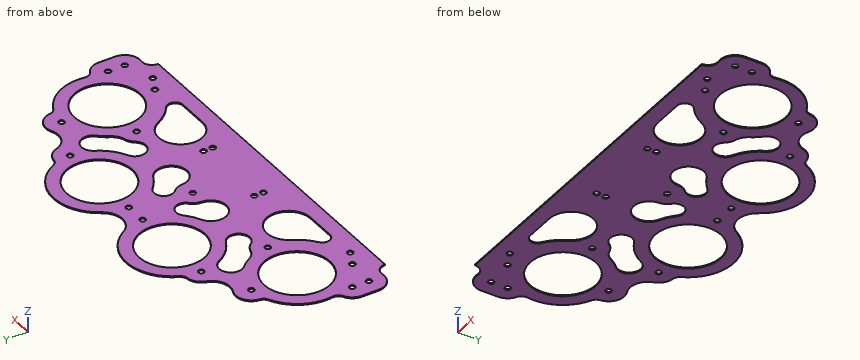
```python
from build123d import *

# Parameters (mm, degrees)
MODEL_R            = 21.5
MODEL_R_2          = 1.89865
BASE_FLANGE1_DEPTH = 0.7


# Sheet-metal steps are written as plain solids
with BuildPart() as part:
    # Model → Base-Flange1 (new body)
    with BuildSketch(Plane.XY):
        with BuildLine():
            Line((-134.72553251, -2.711313899), (-134.72553251, 8.193532943))
            ThreePointArc((-134.72553251, 8.193532943), (-133.25770932, 13.409082664), (-129.285140732, 17.093531418))
            ThreePointArc((-129.285140732, 17.093531418), (-127.122461212, 19.249115875), (-126.616601885, 22.260400219))
            ThreePointArc((-126.616601885, 22.260400219), (-123.404934832, 40.6646253), (-109.924644657, 53.599542498))
            ThreePointArc((-109.924644657, 53.599542498), (-107.998724055, 55.233004005), (-107.116719879, 57.599316598))
            ThreePointArc((-107.116719879, 57.599316598), (-101.974015213, 65.474503584), (-92.575264278, 65.83431216))
            ThreePointArc((-92.575264278, 65.83431216), (-82.894170466, 65.746450056), (-76.506575672, 73.021745919))
            ThreePointArc((-76.506575672, 73.021745919), (-73.335376859, 77.830552746), (-68.037655249, 80.092249178))
            ThreePointArc((-68.037655249, 80.092249178), (-65.683638934, 80.995038824), (-64.06940128, 82.931700578))
            ThreePointArc((-64.06940128, 82.931700578), (-38.361840541, 100.119815012), (-11.129181755, 85.467434576))
            ThreePointArc((-11.129181755, 85.467434576), (0.155495187, 79.042938382), (11.440172129, 85.467434576))
            ThreePointArc((11.440172129, 85.467434576), (38.672830915, 100.119815012), (64.380391655, 82.931700578))
            ThreePointArc((64.380391655, 82.931700578), (65.994629309, 80.995038824), (68.348645623, 80.092249178))
            ThreePointArc((68.348645623, 80.092249178), (73.646367234, 77.830552746), (76.817566047, 73.021745919))
            ThreePointArc((76.817566047, 73.021745919), (83.205160841, 65.746450057), (92.886254653, 65.83431216))
            ThreePointArc((92.886254653, 65.83431216), (102.285005587, 65.474503584), (107.427710253, 57.599316599))
            ThreePointArc((107.427710253, 57.599316599), (108.309714429, 55.233004005), (110.235635031, 53.599542498))
            ThreePointArc((110.235635031, 53.599542498), (123.715925206, 40.6646253), (126.92759226, 22.260400219))
            ThreePointArc((126.92759226, 22.260400219), (127.433451587, 19.249115875), (129.596131107, 17.093531418))
            ThreePointArc((129.596131107, 17.093531418), (133.568699694, 13.409082664), (135.036522885, 8.193532943))
            Line((135.036522885, 8.193532943), (135.036522885, -2.711313899))
            ThreePointArc((135.036522885, -2.711313899), (131.562361662, -10.288478821), (123.553837233, -12.600785232))
            ThreePointArc((123.553837233, -12.600785232), (118.393911689, -14.090613855), (116.155495187, -18.972612677))
            Line((116.155495187, -18.972612677), (-115.844504813, -18.972612677))
            ThreePointArc((-115.844504813, -18.972612677), (-118.082921315, -14.090613855), (-123.242846859, -12.600785232))
            ThreePointArc((-123.242846859, -12.600785232), (-131.251371287, -10.288478821), (-134.72553251, -2.711313899))
        make_face()
        with Locations((97.237534512, 26.561617598)):
            Circle(MODEL_R, mode=Mode.SUBTRACT)
        with Locations((37.237534512, 70.154169278)):
            Circle(MODEL_R, mode=Mode.SUBTRACT)
        with Locations((-36.926544138, 70.154169278)):
            Circle(MODEL_R, mode=Mode.SUBTRACT)
        with Locations((-96.926544138, 26.561617598)):
            Circle(MODEL_R, mode=Mode.SUBTRACT)
        with Locations((-66.926544138, 26.561617598)):
            Circle(MODEL_R_2, mode=Mode.SUBTRACT)
        with Locations((-96.926544138, 56.561617598)):
            Circle(MODEL_R_2, mode=Mode.SUBTRACT)
        with Locations((-66.926544138, 70.154169278)):
            Circle(MODEL_R_2, mode=Mode.SUBTRACT)
        with Locations((-6.926544138, 70.154169278)):
            Circle(MODEL_R_2, mode=Mode.SUBTRACT)
        with Locations((7.237534512, 70.154169278)):
            Circle(MODEL_R_2, mode=Mode.SUBTRACT)
        with Locations((67.237534512, 70.154169278)):
            Circle(MODEL_R_2, mode=Mode.SUBTRACT)
        with Locations((67.237534512, 26.561617598)):
            Circle(MODEL_R_2, mode=Mode.SUBTRACT)
        with Locations((97.237534512, 56.561617598)):
            Circle(MODEL_R_2, mode=Mode.SUBTRACT)
        with Locations((31.205495187, 5.741109522)):
            Circle(MODEL_R_2, mode=Mode.SUBTRACT)
        with Locations((31.205495187, -0.258890478)):
            Circle(MODEL_R_2, mode=Mode.SUBTRACT)
        with Locations((-20.594504813, 5.741109522)):
            Circle(MODEL_R_2, mode=Mode.SUBTRACT)
        with Locations((-20.594504813, -0.258890478)):
            Circle(MODEL_R_2, mode=Mode.SUBTRACT)
        with Locations((106.155495187, -8.972612677)):
            Circle(MODEL_R_2, mode=Mode.SUBTRACT)
        with Locations((96.155495187, -3.972612677)):
            Circle(MODEL_R_2, mode=Mode.SUBTRACT)
        with Locations((-95.844504813, -8.972612677)):
            Circle(MODEL_R_2, mode=Mode.SUBTRACT)
        with Locations((-105.844504813, -3.972612677)):
            Circle(MODEL_R_2, mode=Mode.SUBTRACT)
        with Locations((0.155495187, 32.741109522)):
            Circle(MODEL_R_2, mode=Mode.SUBTRACT)
        with Locations((125.036522885, 8.193532943)):
            Circle(MODEL_R_2, mode=Mode.SUBTRACT)
        with Locations((125.036522885, -2.711313899)):
            Circle(MODEL_R_2, mode=Mode.SUBTRACT)
        with Locations((-124.72553251, 8.193532943)):
            Circle(MODEL_R_2, mode=Mode.SUBTRACT)
        with Locations((-124.72553251, -2.711313899)):
            Circle(MODEL_R_2, mode=Mode.SUBTRACT)
        with BuildLine():
            Line((-55.174396268, -8.972612677), (-75.044791575, -8.972612677))
            ThreePointArc((-75.044791575, -8.972612677), (-79.805084567, -5.502191259), (-77.957288455, 0.091543068))
            ThreePointArc((-77.957288455, 0.091543068), (-72.228077848, 5.337026443), (-67.904131763, 11.790121847))
            ThreePointArc((-67.904131763, 11.790121847), (-42.997191019, 12.776991486), (-55.174396268, -8.972612677))
        make_face(mode=Mode.SUBTRACT)
        with BuildLine():
            Line((75.35578195, -8.972612677), (55.485386642, -8.972612677))
            ThreePointArc((55.485386642, -8.972612677), (43.308181393, 12.776991486), (68.215122138, 11.790121847))
            ThreePointArc((68.215122138, 11.790121847), (72.539068222, 5.337026444), (78.26827883, 0.091543068))
            ThreePointArc((78.26827883, 0.091543068), (80.116074941, -5.502191258), (75.35578195, -8.972612677))
        make_face(mode=Mode.SUBTRACT)
        with BuildLine():
            ThreePointArc((-70.676544138, 41.085305146), (-72.916715678, 44.548505526), (-75.610729677, 47.671711247))
            ThreePointArc((-75.610729677, 47.671711247), (-74.68821375, 59.040915165), (-63.59038518, 56.405002726))
            ThreePointArc((-63.59038518, 56.405002726), (-57.854979641, 48.659970354), (-49.959750183, 43.133148939))
            ThreePointArc((-49.959750183, 43.133148939), (-47.569458742, 32.101093782), (-58.851767466, 32.46059901))
            ThreePointArc((-58.851767466, 32.46059901), (-61.310927531, 34.835966522), (-64.426544138, 36.244075963))
            ThreePointArc((-64.426544138, 36.244075963), (-68.050268495, 38.020840178), (-70.676544138, 41.085305146))
        make_face(mode=Mode.SUBTRACT)
        with BuildLine():
            ThreePointArc((-6.784417864, 39.940943329), (-6.664317076, 48.950582141), (-15.674709396, 48.979667628))
            ThreePointArc((-15.674709396, 48.979667628), (-19.687101522, 45.602150659), (-24.226386782, 42.975022802))
            ThreePointArc((-24.226386782, 42.975022802), (-25.600244312, 25.408712194), (-9.830574629, 33.268754878))
            ThreePointArc((-9.830574629, 33.268754878), (-8.941303628, 36.894210931), (-6.784417864, 39.940943329))
        make_face(mode=Mode.SUBTRACT)
        with BuildLine():
            ThreePointArc((10.141565004, 33.268754878), (25.911234687, 25.408712194), (24.537377157, 42.975022802))
            ThreePointArc((24.537377157, 42.975022802), (19.998091896, 45.602150659), (15.98569977, 48.979667628))
            ThreePointArc((15.98569977, 48.979667628), (6.975307449, 48.950582143), (7.095408238, 39.940943329))
            ThreePointArc((7.095408238, 39.940943329), (9.252294003, 36.894210931), (10.141565004, 33.268754878))
        make_face(mode=Mode.SUBTRACT)
        with BuildLine():
            ThreePointArc((64.737534512, 36.244075963), (68.361258869, 38.020840178), (70.987534512, 41.085305146))
            ThreePointArc((70.987534512, 41.085305146), (73.227706053, 44.548505526), (75.921720052, 47.671711247))
            ThreePointArc((75.921720052, 47.671711247), (74.999204125, 59.040915165), (63.901375554, 56.405002726))
            ThreePointArc((63.901375554, 56.405002726), (58.165970015, 48.659970354), (50.270740558, 43.133148939))
            ThreePointArc((50.270740558, 43.133148939), (47.880449116, 32.101093782), (59.16275784, 32.46059901))
            ThreePointArc((59.16275784, 32.46059901), (61.621917905, 34.835966522), (64.737534512, 36.244075963))
        make_face(mode=Mode.SUBTRACT)
    extrude(amount=-BASE_FLANGE1_DEPTH)


solid = part.part
```
Part model, mm, in its own coordinate system. Give positions to 0.01 mm unless a question says otherwise; leave off trailing zeros. Write each loop counter-clockwise with the first axis right and the second up, starting at its lowest first coordinate (ties: lowest second). Pieces come first, ordered by that corner, then holes. Notation, with made-up numbers: (-37, 45.25) -> (22, 45.25) arc R10 cw to (22, 49.25) -> close; hole circle Ø3 at (55.25, 63.5). An arc over 180 degrees is marked (long way). Put each result on its own line as item: value. Start each with the question number.
Item 1: Cut at A-A (x = 36.5). List the corners of the cut face in (y, z), then the cut area to 3 significant figures.
Item 2: Wall check: L1, parallel to X at y = 4, z = -0.45; L2, parallel to Y at x = 62.5, z = -0.3; L3, parallel to Y at x = -23.5, z = -0.45. Give the ranges that are in metal, low to high. Write a range as [from, to].
Item 3: Cut at C-C (x = -86). List the corners of the cut face in (y, z).
Item 4: Cut at B-B (z = -0.5). State how many separate pieces and enclosed holes the cut face has, then the cut area to 3 significant figures.
Answer list:
1. outline: (-18.97, -0.7) -> (48.67, -0.7) -> (48.67, 0) -> (-18.97, 0) -> close; (91.64, -0.7) -> (100.15, -0.7) -> (100.15, 0) -> (91.64, 0) -> close
1. area: 53.3 mm2
2. L1: x = [-134.73, -73.44], [-40.95, -21.35], [-19.84, 30.45], [31.96, 41.26], [73.75, 135.04]
2. L2: y = [-18.97, -8.97], [17.75, 35.37], [53.97, 86.33]
2. L3: y = [-18.97, 24.33], [43.33, 53.36], [86.95, 96.98]
3. outline: (-18.97, -0.7) -> (8.05, -0.7) -> (8.05, 0) -> (-18.97, 0) -> close; (45.08, -0.7) -> (64.85, -0.7) -> (64.85, 0) -> (45.08, 0) -> close
4. separate pieces: 1
4. enclosed holes: 31
4. area: 15,300 mm2
